Geometry: see drawing. Coordinates: mm, zero at the bounding-box minimum. Coordinates: 2 decimals unless noted, no trailing zeros. Write each loop counter-clockwise with the first axis right and the second up, starting at its lowest first coordinate (ties: lowest second). Pieces come first, ordered by that corner, then holes.
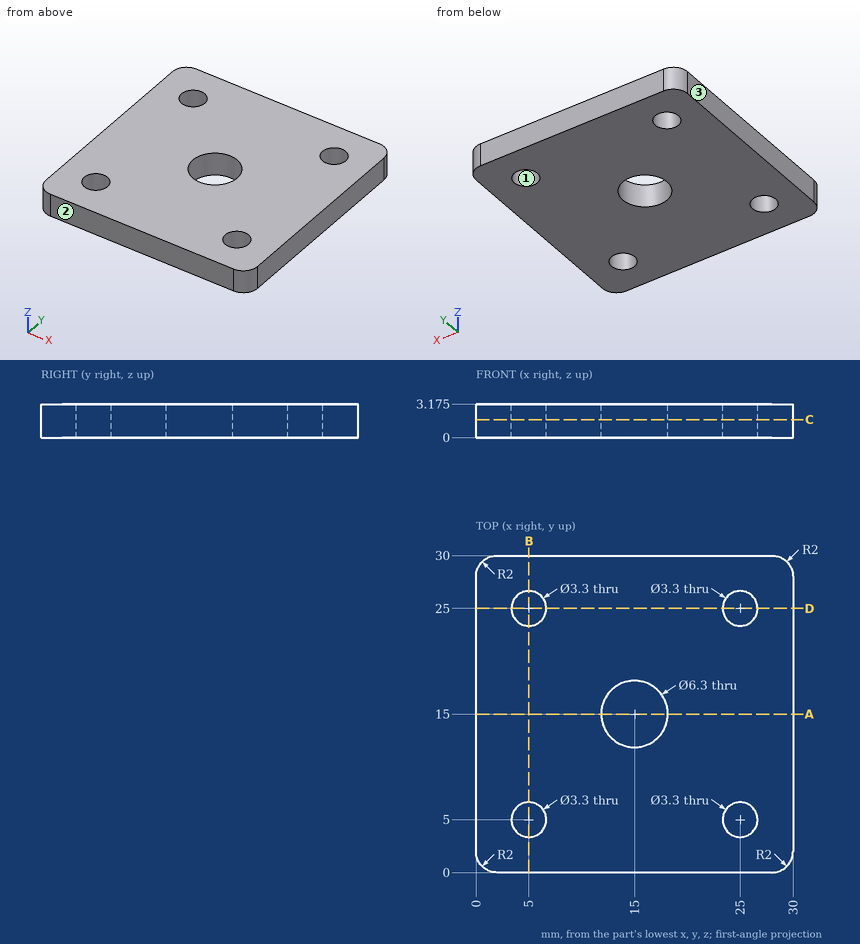
Item 1: Section B-B, the plane x = 5. Output: boundary loops of the cut face in (y, z) (3 decimals), plus the area to 3 significant figures.
Derived:
outline: (0, 0) - (3.35, 0) - (3.35, 3.175) - (0, 3.175) - close; (6.65, 0) - (23.35, 0) - (23.35, 3.175) - (6.65, 3.175) - close; (26.65, 0) - (30, 0) - (30, 3.175) - (26.65, 3.175) - close
area: 74.3 mm2
Item 2: Pull-direction query (X, two-part tool) for the marked faces 1, 2 and 3; classes: released by +X, released by -X, zero draft, split by the parting line, or undercut.
Derived:
face 1: undercut
face 2: zero draft
face 3: released by -X
Item 3: Pin query (flat end, axial travel): pin 1 (2.5 mm diameter, centred on x = 25, y = 25, fed in from -Z). Return the tip coordinate at first contact, or that it passes through.
Derived:
pin 1: passes through
Item 4: Section C-C, the plane z = 1.7. Output: boundary loops of the cut face in (x, y), plus the area to 3 significant figures.
Derived:
outline: (0, 2) arc R2 ccw to (2, 0) - (28, 0) arc R2 ccw to (30, 2) - (30, 28) arc R2 ccw to (28, 30) - (2, 30) arc R2 ccw to (0, 28) - close; hole circle Ø3.3 at (5, 5); hole circle Ø3.3 at (5, 25); hole circle Ø6.3 at (15, 15); hole circle Ø3.3 at (25, 5); hole circle Ø3.3 at (25, 25)
area: 831 mm2
Item 5: Material intervals for probe 1 along X at (y, z) = (25, 0.4); probe 2 along Y at (x, z) = (24.25, 1.05), sorted ascending.
Derived:
probe 1: x = 0 to 3.35, 6.65 to 23.35, 26.65 to 30
probe 2: y = 0 to 3.53, 6.47 to 23.53, 26.47 to 30
Item 6: Section A-A, the plane y = 15. Output: boundary loops of the cut face in (x, z) (3 decimals).
Derived:
outline: (0, 0) - (11.85, 0) - (11.85, 3.175) - (0, 3.175) - close; (18.15, 0) - (30, 0) - (30, 3.175) - (18.15, 3.175) - close
